Autodesk Inventor part; units mm, degrees
ref_plane "YZ Plane" through (0, 0, 0) normal (1, 0, 0) x (0, 1, 0)
ref_plane "XZ Plane" through (0, 0, 0) normal (0, 1, 0) x (-1, 0, 0)
ref_plane "XY Plane" through (0, 0, 0) normal (0, 0, 1) x (1, 0, 0)
sketch "Sketch1" plane through (0, 0, 0) normal (0, 0, 1) x (1, 0, 0)
  line L0 (0, 0) -> (100, 0)
  line L1 (100, 0) -> (100, 8.85)
  line L2 (87.85, 12) -> (12.15, 12)
  line L3 (0, 8.85) -> (0, 0)
  line L4 (12.15, 12) -> (12.15, 8.85)
  line L5 (12.15, 8.85) -> (0, 8.85)
  line L6 (87.85, 12) -> (87.85, 8.85)
  line L7 (87.85, 8.85) -> (100, 8.85)
  dimension "d6" = 100
  dimension "d7" = 3.15
  dimension "d8" = 3.15
  dimension "d9" = 12.15
  dimension "d10" = 12.15
  dimension "d11" = 8.85
  dimension "d12" = 8.85
  dimension "d13" = 12
extrude "Extrusion1" add sketch "Sketch1" along normal blind 6
sketch "Sketch2" plane through (0, 0, 0) normal (0, 0, -1) x (-1, 0, 0)
  line L0 (-87.85, 12) -> (-12.15, 12)
  line L1 (0, 0) -> (-100, 0)
  line L2 (-87.85, 12) -> (-12, 12)
  line L3 (-12, 12) -> (-12, 0)
  line L4 (-12, 0) -> (-87.85, 0)
  line L5 (-87.85, 0) -> (-87.85, 12)
extrude "Extrusion2" add sketch "Sketch2" along normal blind 6
sketch "Sketch3" plane through (0, 0, 0) normal (0, 0, -1) x (-1, 0, 0)
  circle A0 centre (-6, 4.35) radius 1.725
  line L0 (-12, 8.85) -> (0, 8.85)
  line L1 (0, 8.85) -> (0, 0)
  circle A1 centre (-94, 4.5) radius 1.725
  line L2 (-87.85, 0) -> (-100, 0)
  line L3 (-100, 0) -> (-100, 8.85)
  point P0 (-12, 9)
  dimension "d18" = 3.45
  dimension "d19" = 4.5
  dimension "d20" = 6
  dimension "d21" = 3.45
  dimension "d22" = 4.5
  dimension "d23" = 6
extrude "Extrusion3" cut sketch "Sketch3" against normal blind 4
sketch "Sketch4" plane through (0, 0, 6) normal (0, 0, 1) x (1, 0, 0)
  circle A0 centre (6, 4.35) radius 3
  line L0 (12.15, 8.85) -> (0, 8.85)
  line L1 (0, 8.85) -> (0, 0)
  circle A1 centre (94, 4.5) radius 1.725
  circle A2 centre (94, 4.5) radius 3
  dimension "d26" = 6
  dimension "d27" = 4.5
  dimension "d28" = 6
  dimension "d29" = 6
extrude "Extrusion4" cut sketch "Sketch4" against normal blind 2 contours A0 | A1 | A2
sketch "Sketch5" plane through (87.85, 0, 0) normal (0, -1, 0) x (1, 0, 0)
  point P0 (-87.85, 0)
sketch "Sketch6" plane through (0, 0, 0) normal (0, 0, -1) x (-1, 0, 0)
  line L0 (0, 0) -> (-100, 0)
  line L1 (-12.15, 8.85) -> (0, 8.85)
  line L2 (0, 0) -> (0, 8.85)
  line L3 (-12.15, 8.85) -> (-12, 8.85)
  line L4 (0, 8.85) -> (-12, 8.85)
  line L5 (-12, 0) -> (-12, 12)
  line L6 (-12, 8.85) -> (-12, 0)
  line L7 (-12, 0) -> (0, 0)
  line L8 (-100, 0) -> (-100, 8.85)
  line L9 (-100, 0) -> (-87.85, 0)
  line L10 (-87.85, 0) -> (-87.85, 8.85)
  line L11 (-87.85, 0) -> (-87.85, 8.85)
  line L12 (-87.85, 8.85) -> (-100, 8.85)
  line L13 (-100, 8.85) -> (-100, 0)
  dimension "d33" = 12.15
extrude "Extrusion5" cut sketch "Sketch6" against normal blind 0.15
sketch "Sketch7" plane through (12, 8.85, 0) normal (-1, 0, 0) x (0, 0, 1)
  line L0 (0, 3.15) -> (0, 0)
  line L1 (0, 3.15) -> (0, 0)
  line L2 (0.15, 0) -> (6, 0)
  line L3 (0, 0) -> (0.15, 0)
  line L4 (0.15, 0) -> (0.15, -8.85)
  line L5 (0.15, 0) -> (0.15, -8.85)
  line L6 (0.15, -8.85) -> (-6, -8.85)
  line L7 (0.15, -8.85) -> (-6, -8.85)
  line L8 (-6, -8.85) -> (-6, 3.15)
  line L9 (0, 3.15) -> (6, 3.15)
  line L10 (-6, 3.15) -> (0, 3.15)
  point P0 (0, -8.85)
sketch "Sketch8" plane through (12.15, 12, 6) normal (0, 1, 0) x (1, 0, 0)
  line L0 (0, 6) -> (0, 0)
  line L1 (75.7, 12) -> (-0.15, 12)
  line L2 (0, 6) -> (-0.15, 6)
  line L3 (-0.15, 6) -> (-0.15, 12)
  line L4 (-0.15, 12) -> (0, 12)
  line L5 (0, 12) -> (0, 6)
  point P0 (-12.15, 6)
extrude "Extrusion6" cut sketch "Sketch7" against normal blind 0.15
fillet "Fillet2" radius 1.5 2 edges at (50, 12, 6) (50, 12, -6)
equation "\"d8\" = d7"
equation "\"d10\" = d9"
equation "\"d12\" = d11"
properties part number "beam10cmVer2"
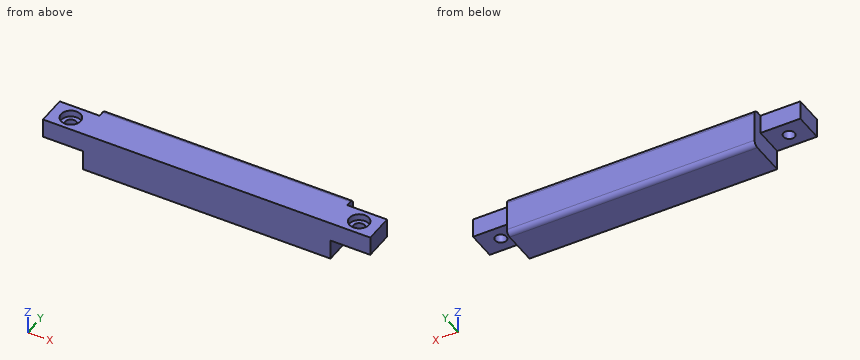
Geometry: final body of the model. Coordinates: model frame, mm. Coordinates: 2 decimals unless noted, no trailing zeros. Order: outer loops, then holes, each group sorted by start corner. A loop starts at its lowest first (then second) coordinate and runs counter-clockwise, first axis right, second up. Notation, with made-up numbers: (63.5, 54.25) -> (81.5, 54.25) arc R5 cw to (81.5, 60.25) -> close; hole circle Ø10 at (-5, -24.75). An arc over 180 degrees is marked (long way). Answer in a Markdown table with one row per item.
Item 1: Section A-A on x = 94. Output: boundary loops of the cut face in (y, z) (3 decimals).
Return value:
| item | result |
|---|---|
| outline | (0, 0.15) -> (2.775, 0.15) -> (2.775, 4) -> (1.5, 4) -> (1.5, 6) -> (0, 6) -> close; (6.225, 0.15) -> (8.85, 0.15) -> (8.85, 6) -> (7.5, 6) -> (7.5, 4) -> (6.225, 4) -> close |
Item 2: Ray query, L1, parallel to Y at x = 6, z = 5.5; L2, parallel to Y at x = 94, z = 3.2 (3 decimals); L3, parallel to X at y = 11.25, z = -5.5. Return the intervals inside material, ascending.
Return value:
| item | result |
|---|---|
| L1 | y = 0 to 1.35, 7.35 to 8.85 |
| L2 | y = 0 to 2.775, 6.225 to 8.85 |
| L3 | x = 12.15 to 87.85 |
Item 3: Contact query for flat-ended pins moving along their axis: P1, Ø1.8, axis at x = 95.5, y = 4.5, coming from the +Z side; P2, Ø4.5, axis at x = 93, z = 4.5, coming from the +Y side; P3, Ø3, axis at y = 10, z = -3, coming from the -X side. Output: stop coordinate, or through.
Return value:
| item | result |
|---|---|
| P1 | stops at z = 4 |
| P2 | stops at y = 8.85 |
| P3 | stops at x = 12.15 |
Item 4: Section B-B on z = 1. Output: boundary loops of the cut face in (x, y) (3 decimals).
Return value:
| item | result |
|---|---|
| outline | (0, 0) -> (100, 0) -> (100, 8.85) -> (87.85, 8.85) -> (87.85, 12) -> (12.15, 12) -> (12.15, 8.85) -> (0, 8.85) -> close; hole circle Ø3.45 at (6, 4.35); hole circle Ø3.45 at (94, 4.5) |
Item 5: Section C-C on z = -3. Output: boundary loops of the cut face in (x, y).
Return value:
| item | result |
|---|---|
| outline | (12.15, 0) -> (87.85, 0) -> (87.85, 12) -> (12.15, 12) -> close |
